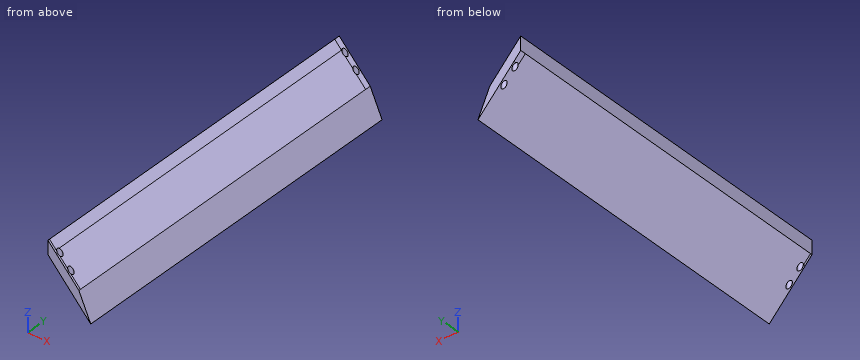
Autodesk Inventor part; units mm, degrees
ref_plane "YZ Plane" through (0, 0, 0) normal (1, 0, 0) x (0, 1, 0)
ref_plane "XZ Plane" through (0, 0, 0) normal (0, 1, 0) x (-1, 0, 0)
ref_plane "XY Plane" through (0, 0, 0) normal (0, 0, 1) x (1, 0, 0)
sketch "Sketch1" plane through (0, 0, 0) normal (0, 1, 0) x (-1, 0, 0)
  line L0 (20.0075, 12.0668) -> (-3.1128, -12.9332)
  line L1 (-3.1128, -12.9332) -> (20.0075, 12.0668)
  line L2 (-3.1128, -17.9332) -> (-3.1128, -12.9332)
  line L3 (-3.1128, -17.9332) -> (-14.7232, -17.9332)
  line L4 (-3.1128, -17.9332) -> (-3.1128, -12.9332)
  line L5 (-3.1128, -17.9332) -> (-8.918, -17.9332)
  arc A0 (-14.7232, -17.9332) -> (-3.1128, -12.9332) centre (-21.6099, 14.0384) ccw
  line L6 (-14.7232, -17.9332) -> (20.7671, -17.9332)
  line L7 (20.0075, 12.0668) -> (20.0075, -17.9332)
  line L8 (20.0075, 12.0668) -> (20.0075, 17.0668)
  line L9 (16.3366, 15.4617) -> (-8.1128, -10.9755)
  line L10 (16.3366, 15.4617) -> (20.0075, 19.431)
  line L11 (20.0075, 19.431) -> (20.0075, 15.7489)
  line L12 (-14.7232, -17.9332) -> (-8.1128, -10.9755)
  point P0 (0, 0)
  dimension "d0" = 5
  dimension "d1" = 5
extrude "Extrusion1" add sketch "Sketch1" along normal blind 186.69 contours L0 A0 L12 L9 L10 L11 L8
sketch "Sketch2" plane through (0, 0, 0) normal (0, -1, 0) x (1, 0, 0)
  line L0 (3.1128, -12.9332) -> (-20.0075, 12.0668)
  line L1 (-20.0075, 12.0668) -> (-16.3304, 12.0668)
  line L2 (-16.3304, 12.0668) -> (-16.3304, -0.4332)
  line L3 (-16.3304, -0.4332) -> (-20.0075, -0.4332)
  line L4 (-20.0075, -0.4332) -> (-20.0075, 12.0668)
  circle A0 centre (-18.1689, 1.5735) radius 1.35
  circle A1 centre (-18.1689, 5.8168) radius 1.35
  point P0 (0, 0)
  point P1 (-16.3304, 8.0908)
  dimension "d4" = 2.7
  dimension "d5" = 2.7
extrude "Extrusion2" add sketch "Sketch2" along normal blind 3 contours L2 L3 L4 L0
sketch "Sketch3" plane through (0, 0, 0) normal (0, -1, 0) x (1, 0, 0)
  line L0 (-20.0075, 12.0668) -> (-20.0075, 19.431)
  line L1 (3.1128, -12.9332) -> (-20.0075, 12.0668)
  line L2 (-20.0075, 19.431) -> (-20.0075, 12.0668)
  line L3 (-20.0075, 12.0668) -> (3.1128, -12.9332)
  arc A0 (3.1128, -12.9332) -> (14.7232, -17.9332) centre (21.6099, 14.0384) ccw
  arc A1 (3.1128, -12.9332) -> (14.6054, -17.9076) centre (21.6099, 14.0384) ccw
  line L4 (8.1128, -10.9755) -> (14.7232, -17.9332)
  line L5 (8.1128, -10.9755) -> (14.7232, -17.9332)
  line L6 (-20.0075, 19.431) -> (8.1128, -10.9755)
  point P0 (0, 0)
extrude "Extrusion3" add sketch "Sketch3" along normal blind 3
sketch "Sketch4" plane through (0, 186.69, 0) normal (0, 1, 0) x (1, 0, 0)
  circle A0 centre (-18.1689, -5.8168) radius 1.35
  circle A1 centre (-18.1689, -1.5735) radius 1.35
  line L0 (-20.0075, -19.431) -> (-20.0075, 0.4332)
  line L1 (-20.0075, 0.4332) -> (-16.3304, 0.4332)
  line L2 (-16.3304, 0.4332) -> (-16.3304, -8.0908)
  line L3 (8.1128, 10.9755) -> (14.7232, 17.9332)
  line L4 (14.7232, 17.9332) -> (8.1128, 10.9755)
  line L5 (-20.0075, -19.431) -> (8.1128, 10.9755)
  line L6 (8.1128, 10.9755) -> (-20.0075, -19.431)
  line L7 (-20.0075, -19.431) -> (-20.0075, 0.4332)
  line L8 (-20.0075, 0.4332) -> (-16.3304, 0.4332)
  line L9 (-20.0075, 0.4332) -> (-16.3304, 0.4332)
  line L10 (-16.3304, 0.4332) -> (-16.3304, -8.0908)
  line L11 (3.1128, 12.9332) -> (-20.0075, -12.0668)
  line L12 (-16.3304, -8.0908) -> (3.1128, 12.9332)
  arc A2 (14.7232, 17.9332) -> (3.1128, 12.9332) centre (21.6099, -14.0384) ccw
  arc A3 (-20.0075, -12.0668) -> (-20.0075, -10.5639) centre (-20.8201, -11.3154) ccw
  line L13 (-16.3304, 0.4332) -> (-20.0075, 0.4332)
  point P0 (0, 0)
extrude "Extrusion4" add sketch "Sketch4" along normal blind 3
sketch "Sketch5" plane through (0, 189.69, 0) normal (0, 1, 0) x (1, 0, 0)
  line L0 (-16.3304, -8.0908) -> (3.1128, 12.9332)
  line L1 (3.1128, 12.9332) -> (3.1128, 4.2571)
  line L2 (3.1128, 4.2571) -> (16.783, 4.2571)
  line L3 (16.783, 4.2571) -> (16.783, 22.684)
  line L4 (16.783, 22.684) -> (3.1128, 22.684)
  line L5 (3.1128, 22.684) -> (3.1128, 12.9332)
  point P0 (0, 0)
extrude "Extrusion5" cut sketch "Sketch5" against normal blind 200
sketch "Sketch6" plane through (0, 189.69, 0) normal (0, 1, 0) x (1, 0, 0)
  line L0 (3.1128, 12.9332) -> (-16.3304, -8.0908)
  line L1 (3.1128, 12.9332) -> (-3.2785, -1.3419)
  line L2 (-20.0075, -19.431) -> (3.1128, 5.569)
  line L3 (3.1128, 5.569) -> (3.1128, 12.9332)
  line L4 (3.1128, 5.569) -> (-3.2785, -1.3419)
  line L5 (3.1128, 5.569) -> (3.1128, 12.9332)
  point P0 (0, 0)
extrude "Extrusion6" cut sketch "Sketch6" against normal blind 200
sketch "Sketch7" plane through (0, -3, 0) normal (0, -1, 0) x (1, 0, 0)
  line L0 (-16.3304, 8.0908) -> (-16.3304, -0.4332)
  line L1 (-16.3304, 8.0908) -> (-20.0075, 12.0668)
  line L2 (-16.3304, 8.0908) -> (-20.0075, 12.0668)
  line L3 (-20.0075, -0.4332) -> (-20.0075, 19.431)
  line L4 (-20.0075, 12.0668) -> (-20.0075, -0.4332)
  line L5 (-16.3304, -0.4332) -> (-20.0075, -0.4332)
  line L6 (-20.0075, -0.4332) -> (-16.3304, -0.4332)
  line L7 (-16.3304, -0.4332) -> (-16.3304, 8.0908)
  point P0 (0, 0)
extrude "Extrusion7" cut sketch "Sketch7" against normal blind 222
sketch "Sketch8" plane through (-20.0075, -3, 19.431) normal (0.7341688, 0, 0.678967) x (0.678967, 0, -0.7341688)
  line L0 (0, 0) -> (0, 192.69)
  line L1 (0, 192.69) -> (0, 2)
  line L2 (0, 2) -> (41.2163, 2)
  line L3 (41.2163, 2) -> (41.2163, -1.239)
  line L4 (41.2163, -1.239) -> (0, -1.239)
  line L5 (0, -1.239) -> (0, 2)
  point P0 (27.85, 3)
  dimension "d18" = 190.69
extrude "Extrusion8" cut sketch "Sketch8" against normal blind 222
sketch "Sketch9" plane through (0, 0, 0) normal (0, 0, 1) x (1, 0, 0)
  circle A0 centre (-15.245, 1.0241) radius 1.35
  line L0 (-20.0075, -1) -> (-20.0075, 189.69)
  line L1 (-20.0075, 94.345) -> (7.4426, 94.345)
  circle A1 centre (-9.2868, 1.0241) radius 1.35
  circle A2 centre (-15.245, 187.6659) radius 1.35
  circle A3 centre (-9.2868, 187.6659) radius 1.35
  point P0 (0, 0)
  dimension "d21" = 2.7
  dimension "d22" = 2.7
extrude "Extrusion9" cut sketch "Sketch9" along normal mid plane 222
sketch "Sketch10" plane through (0, 0, 0) normal (0, 0, 1) x (1, 0, 0)
  circle A0 centre (-15.245, 1.0241) radius 1.35
  circle A1 centre (-15.245, 1.0241) radius 1.35
  circle A2 centre (-9.2868, 1.0241) radius 1.35
  circle A3 centre (-9.2868, 1.0241) radius 1.35
  circle A4 centre (-15.245, 187.6659) radius 1.35
  circle A5 centre (-15.245, 187.6659) radius 1.35
  circle A6 centre (-9.2868, 187.6659) radius 1.35
  circle A7 centre (-9.2868, 187.6659) radius 1.35
  line L0 (-16.595, 1.0241) -> (-20.0075, 1.0241)
  line L1 (-20.0075, -1) -> (-20.0075, 189.69)
  line L2 (-20.0075, 1.0241) -> (-20.0075, -1)
  line L3 (-20.0075, -1) -> (-3.2785, -1)
  line L4 (-20.0075, -1) -> (-3.2785, -1)
  point P0 (0, 0)
properties part number "blade"
Can you work these out from the model? Positions are in its coordinate system, mm. Coordinates: 2 decimals unless noted, no trailing zeros. Loops run counter-clockwise (first coordinate to the right, second up) from the corner with the lowest first, then second, coordinate; pieces in that order, holes last. Notation, with made-up numbers: M 13.25,65.5 L 49.25,65.5 A17 ccw 49.25,84.5 Z; hole C -33.75,54.5 d9. An arc over 180 degrees is marked long. Put each result on its own line as item: value. Start each with the question number.
(1) Imagine slicing it at B-B on x = 0.25. List the corners of the cut face in (y, z) for me, and give its area (3 significant figures).
(2) Imagine slicing it at A-A on y = 169. List the corners of the cut face in (x, z) for me, and give its area (3 significant figures).
(3) Will these pins go through, and if not, where does the flat tip stop? pin 1 Ø4.5 at (x, y) = (-15.24, 1.02) entering from -Z; pin 2 Ø4.5 at (x, y) = (-9.29, 187.67) entering from -Z; pin 3 Ø3 at (y, z) = (145.5, 4.5) entering from -X; pin 4 Ø1.6 at (x, y) = (-15.24, 187.67) entering from -Z.
(4) Imagine slicing it at C-C on z = -6. List the corners of the cut face in (x, y) for me.
(5) I need wall thicknesses on probe 1 along Y at (x, z) = (-8.5, 2.5); probe 2 along X at (y, z) = (24.5, -6); probe 3 along Z at (x, y) = (1.5, 122.5). Which ranges of each line are inside material? Lowest first, please.
Worked answers:
1. outline: M -1,-9.84 L 189.69,-9.84 L 189.69,-6.54 L -1,-6.54 Z
1. area: 629 mm2
2. outline: M -20.01,12.07 L 3.11,-12.93 L -3.28,1.34 L -16.34,15.46 L -20.01,19.43 Z
2. area: 147 mm2
3. pin 1: stops at z = 4.48
3. pin 2: stops at z = -1.95
3. pin 3: stops at x = -14.4
3. pin 4: passes through
4. outline: M -3.3,-1 L 0.01,-1 L 0.01,189.69 L -3.3,189.69 Z
5. probe 1: y = -1 to -0.07, 2.12 to 186.57, 188.76 to 189.69
5. probe 2: x = -3.3 to 0.01
5. probe 3: z = -11.19 to -9.33
